Check sheet for the modelled part. Datum: model origin and axes. Units: mm. Coordinates: 2 decimals unless noted, no trailing zeros. Order: outer loops, then holes, each group sorted by start corner. A loop starts at its lowest first (then second) coordinate and runs counter-clockwise, first axis right, second up.
1. Thickness scan on line 1 (X direction, y = 7.75, z = 120); line 2 (Z direction, x = 1, y = 1); line 3 (Z direction, x = -10.5, y = 8.25). Record the ranges inside material, lowest first.
2. Cross-section at B-B (y = 8.25). Count the separate pieces of the cut face and the enclosed holes in it, then the cut area to 3 significant figures.
3. Gauge pin test, flat ends, axial feed: pin 1 Ø1.9 at (x, z) = (0, 160) entering from -Y; pin 2 Ø1.5 at (x, y) = (-16, 6) entering from -Z; pin 3 Ø5 at (x, y) = (-8.5, 2) entering from +Z. Record the tip position at first contact, or that the pin passes through.
4. Cross-section at A-A (z = 120). Enter the section's corners in (x, y).
```python
from build123d import *

# Parameters (mm, degrees)
BOSS_EXTRUDE1_DEPTH = 10
SKETCH3_R           = 1.6
CUT_EXTRUDE1_DEPTH  = 168.182534973
SKETCH4_R           = 1.6
CUT_EXTRUDE2_DEPTH  = 168.182534973
CHAMFER1_SIZE       = 4


with BuildPart() as part:
    # Sketch1 → Boss-Extrude1 (new body)
    with BuildSketch(Plane(origin=(0, 0, 0), x_dir=(1, 0, 0), z_dir=(0, 1, 0))):
        with BuildLine():
            Line((-25, 0), (-25, -140))
            ThreePointArc((-25, -140), (0, -165), (25, -140))
            Line((25, -140), (25, 0))
            ThreePointArc((25, 0), (0, 25), (-25, 0))
        make_face()
    extrude(amount=BOSS_EXTRUDE1_DEPTH)

    # Sketch3 → Cut-Extrude1 (cut, through all)
    with BuildSketch(Plane.XZ):
        with Locations(Location((10.098593171, 0, 0), (0, 0, 270))):
            Circle(SKETCH3_R)
        with Locations(Location((0, 10.098593171, 0), (0, 0, 270))):
            Circle(SKETCH3_R)
        with Locations(Location((0, -10.098593171, 0), (0, 0, 270))):
            Circle(SKETCH3_R)
        with Locations(Location((-10.098593171, 0, 0), (0, 0, 270))):
            Circle(SKETCH3_R)
    extrude(amount=-CUT_EXTRUDE1_DEPTH, mode=Mode.SUBTRACT)

    # Sketch4 → Cut-Extrude2 (cut, through all)
    with BuildSketch(Plane.XZ):
        with Locations(Location((0, 120, 0), (0, 0, 270))):
            Circle(SKETCH4_R)
        with Locations(Location((20, 140, 0), (0, 0, 270))):
            Circle(SKETCH4_R)
        with Locations(Location((0, 160, 0), (0, 0, 270))):
            Circle(SKETCH4_R)
        with Locations(Location((-20, 140, 0), (0, 0, 270))):
            Circle(SKETCH4_R)
    extrude(amount=-CUT_EXTRUDE2_DEPTH, mode=Mode.SUBTRACT)

    # Chamfer1
    # the kernel refuses this chamfer: 4 mm, written as the material it takes off along each edge
    with BuildSketch(Plane(origin=(25, 0, 140), x_dir=(-0.9996219169112968, -0.027495876610586365, 0), z_dir=(0, 0, -1))) as chamfer1_piece_1:
        Polygon((CHAMFER1_SIZE * 0.999621916911, CHAMFER1_SIZE * 0.0274958766106), (-CHAMFER1_SIZE * 0.0274958766106, CHAMFER1_SIZE * 0.999621916911), (0, 0), align=None)
    extrude(amount=140, mode=Mode.SUBTRACT)
    with BuildSketch(Plane(origin=(0, 0, 140), x_dir=(-1, 0, 0), z_dir=(0, 0, -1))) as chamfer1_piece_2:
        Polygon((25, CHAMFER1_SIZE), (25 - CHAMFER1_SIZE, 0), (25, 0), align=None)
    revolve(axis=Axis((0, 0, 140), (0, 1, 0)), revolution_arc=180, mode=Mode.SUBTRACT)
    with BuildSketch(Plane(origin=(-25, 0, 0), x_dir=(-0.027495876610586494, 0.9996219169112968, 0), z_dir=(0, 0, 1))) as chamfer1_piece_3:
        Polygon((CHAMFER1_SIZE * 0.999621916911, -CHAMFER1_SIZE * 0.0274958766106), (-CHAMFER1_SIZE * 0.0274958766106, -CHAMFER1_SIZE * 0.999621916911), (0, 0), align=None)
    extrude(amount=140, mode=Mode.SUBTRACT)
    with BuildSketch(Plane(origin=(0, 0, 0), x_dir=(1, 0, 0), z_dir=(0, 0, 1))) as chamfer1_piece_4:
        Polygon((25, CHAMFER1_SIZE), (25 - CHAMFER1_SIZE, 0), (25, 0), align=None)
    revolve(axis=Axis((0, 0, 0), (0, 1, 0)), revolution_arc=180, mode=Mode.SUBTRACT)


solid = part.part
```
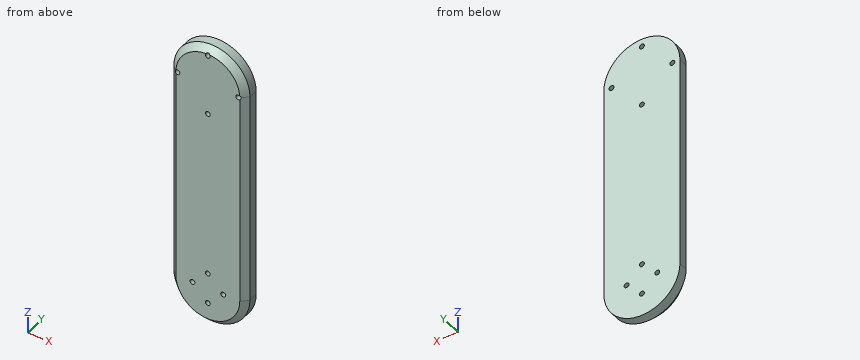
Data:
1. line 1: x = -25 to -1.6, 1.6 to 25
1. line 2: z = -21.98 to -11.35, -8.85 to 8.85, 11.35 to 118.75, 121.25 to 158.75, 161.25 to 161.98
1. line 3: z = -22.69 to -1.55, 1.55 to 162.69
2. separate pieces: 1
2. enclosed holes: 8
2. area: 8,900 mm2
3. pin 1: passes through
3. pin 2: stops at z = -19.81
3. pin 3: stops at z = 164
4. outline: (-25, 4) - (-21, 0) - (-1.6, 0) - (-1.6, 10) - (-25, 10) - close; (1.6, 0) - (21, 0) - (25, 4) - (25, 10) - (1.6, 10) - close
